from build123d import *

# Parameters (mm, degrees)
F0_W     = 38.68904
F0_H     = 70
F1_DEPTH = 60


with BuildPart() as f1:
    # F0 (on Front) → F1 (new body)
    with BuildSketch(Plane.XZ):
        with BuildLine():
            ThreePointArc((-3.082677, 69.82396), (-31.366948, 58.108231), (-43.082677, 29.82396))
            Line((-43.082677, 29.82396), (-43.082677, -20.17604))
            ThreePointArc((-43.082677, -20.17604), (-3.082677, -60.17604), (36.917323, -20.17604))
            Line((36.917323, -20.17604), (36.917323, 29.82396))
            ThreePointArc((36.917323, 29.82396), (25.201594, 58.108231), (-3.082677, 69.82396))
        make_face()
        with Locations((-3.082677, 5.491615)):
            Rectangle(F0_W, F0_H, mode=Mode.SUBTRACT)
    extrude(amount=F1_DEPTH)


solid = f1.part
The model under review builds one solid part; all positions refer to its coordinate system, in mm. A direction names the side the tool comes from. Round coordinates to 2 decimals unless told otherwise and drop trailing zeros. Write each loop counter-clockwise with the first axis right and the second up, starting at its lowest first coordinate (ties: lowest second). Pieces come first, ordered by that corner, then holes. Notation, with made-up numbers: M 11.25,59.25 L 54.25,59.25 A8 cw 54.25,73.25 Z; hole C -24,37.25 d2. An arc over 180 degrees is marked long. Use a Markdown table: item, result. Add a question column.
Q1. We need section D-D, the plane x = -37. State the section outline as (y, z) points, plus the area to 3 significant figures.
Q2. The part is to be moulded in two halves that separate along X. For faces 1 (the face through (-3, -30, 40.492)), 2 (the face through (23, -60, 6)), 3 (the face through (36.917, -30, 4)), say which applies: pulls with the +X half, pulls with the -X half, needs draft (parallel to the pull), parting line crosses it, or undercut.
Q3. We need section B-B, the plane y = -35. State the section outline as (x, z) points, plus the area to 3 significant figures.
Q4. We need section A-A, the plane z = 2. State the section outline as (x, y) points, plus the area to 3 significant figures.
Q5. To check wall thickness, follow line 1 (X direction, y = -26, z = 2.5); line 2 (Z direction, x = 6.5, y = -34); line 3 (Z direction, x = 0, y = -24) (3 decimals). State the ranges of each line that lie inside material, in increasing order.
Q6. Machinability: for faces 4 (the face through (-43.083, -30, 5)), 5 (the face through (-22.427, -30, 5)), which of the approach directions +Z, -Z, +X, -X, +Y, -Y give a long, thin tool a straight path to every point of the face, cutting with its end or side? Answer none if there is none.
Q7. We need section C-C, the plane x = 0. State the section outline as (y, z) points (3 decimals).
Q8. Insertion check: pin 1 (3 mm diameter, centred on x = -20, z = -3, fed in from -Y); pin 2 (12 mm diameter, centred on x = -33.5, y = -30, fed in from +Z); pin 3 (19.5 mm diameter, centred on x = -12.5, y = -16.5, fed in from -Z); pin 4 (2 mm diameter, centred on x = -24, y = -17, fed in from -Z). Each pin has a flat end and moves straight along its axis. Give the tip position at first contact, or say it passes through.
Findings below:
| question | item | result |
|---|---|---|
| 1 | outline | M -60,-41.38 L 0,-41.38 L 0,51.03 L -60,51.03 Z |
| 1 | area | 5,540 mm² |
| 2 | face 1 | undercut |
| 2 | face 2 | needs draft |
| 2 | face 3 | pulls with the +X half |
| 3 | outline | M -43.08,-20.18 A40 ccw 36.92,-20.18 L 36.92,29.82 A40 ccw -3.08,69.82 A40 ccw -43.08,29.82 Z; hole M -22.43,-29.51 L 16.26,-29.51 L 16.26,40.49 L -22.43,40.49 Z |
| 3 | area | 6,320 mm² |
| 4 | outline | M -43.08,-60 L -22.43,-60 L -22.43,0 L -43.08,0 Z; M 16.26,-60 L 36.92,-60 L 36.92,0 L 16.26,0 Z |
| 4 | area | 2,480 mm² |
| 5 | line 1 | x = -43.08 to -22.43, 16.26 to 36.92 |
| 5 | line 2 | z = -59.01 to -29.51, 40.49 to 68.66 |
| 5 | line 3 | z = -60.057 to -29.508, 40.492 to 69.705 |
| 6 | face 4 | +Z, -Z, -X, +Y, -Y |
| 6 | face 5 | +Y, -Y |
| 7 | outline | M -60,-60.057 L 0,-60.057 L 0,-29.508 L -60,-29.508 Z; M -60,40.492 L 0,40.492 L 0,69.705 L -60,69.705 Z |
| 8 | pin 1 | passes through |
| 8 | pin 2 | stops at z = 61.51 |
| 8 | pin 3 | stops at z = -60.18 |
| 8 | pin 4 | stops at z = -54.86 |
